The figure shows three views and two pictorial views of one solid part (mm, origin at its lowest corner). Answer the questions. A direction names the side the tool comes from. Coordinates: 2 decimals unless noted, no trailing zeros. Write each loop counter-clockwise with the first axis right and the second up, starting at its lowest first coordinate (ties: lowest second). Pieces come first, ordered by that corner, then holes.
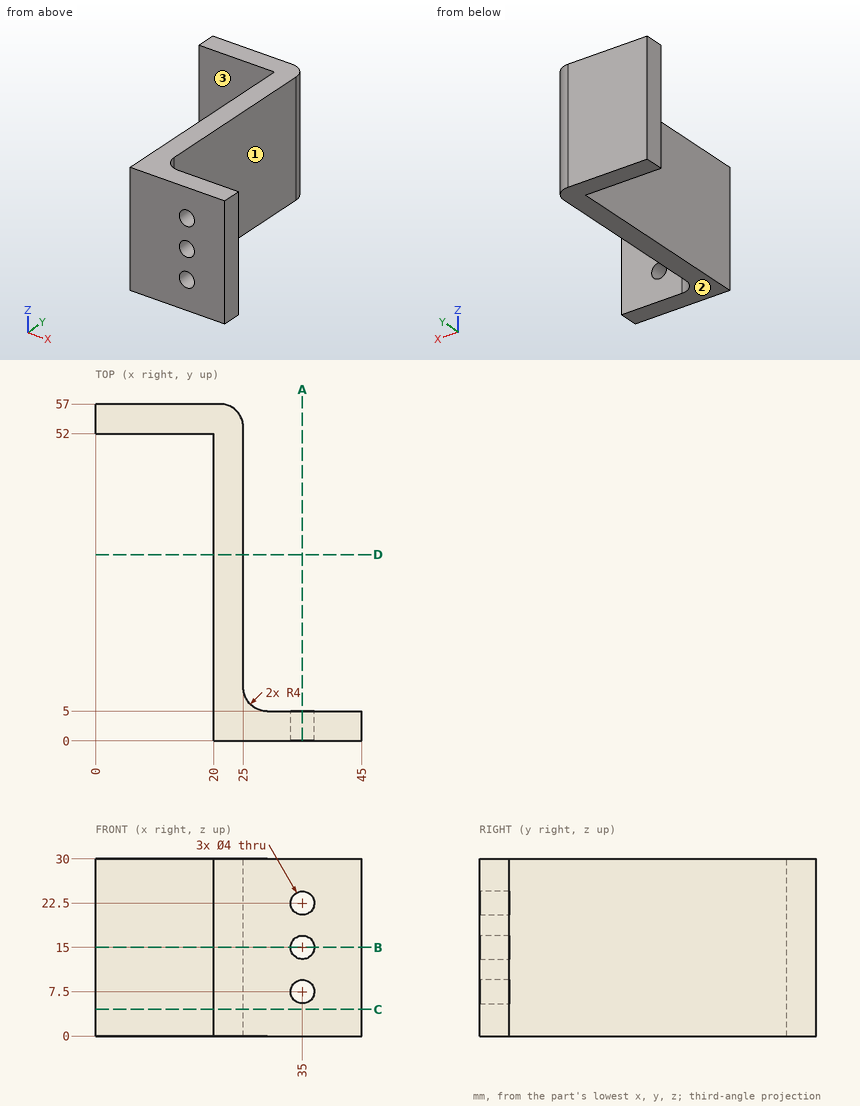
1. Section A-A on x = 35 is taken. Give the vertices of the cut face in (y, z).
Results found:
outline: (0, 0) - (5, 0) - (5, 5.5) - (0, 5.5) - close; (0, 9.5) - (5, 9.5) - (5, 13) - (0, 13) - close; (0, 17) - (5, 17) - (5, 20.5) - (0, 20.5) - close; (0, 24.5) - (5, 24.5) - (5, 30) - (0, 30) - close
2. Flat-ended cylindrical pins translate along their axes: P1, Ø5, axis at y = 48.5, z = 19.5, coming from the +X side; P2, Ø17.5, axis at x = 36, z = 20.5, coming from the +Y side; P3, Ø10, axis at x = 9, z = 17, coming from the -Y side. Find the tip coordinate at first contact, or state that the pin passes through.
Results found:
P1: stops at x = 25
P2: stops at y = 5.4
P3: stops at y = 52
3. Section D-D on y = 31.5 is taken. Give the vertices of the cut face in (x, z), then the cut area to 3 significant figures.
Results found:
outline: (20, 0) - (25, 0) - (25, 30) - (20, 30) - close
area: 150 mm2
4. Section B-B on z = 15 is taken. Give the vertices of the cut face in (x, y).
Results found:
outline: (0, 52) - (20, 52) - (20, 0) - (33, 0) - (33, 5) - (29, 5) arc R4 cw to (25, 9) - (25, 53) arc R4 ccw to (21, 57) - (0, 57) - close; (37, 0) - (45, 0) - (45, 5) - (37, 5) - close
5. Section C-C on z = 4.5 is taken. Give the vertices of the cut face in (x, y), then the cut area to 3 significant figures.
Results found:
outline: (0, 52) - (20, 52) - (20, 0) - (45, 0) - (45, 5) - (29, 5) arc R4 cw to (25, 9) - (25, 53) arc R4 ccw to (21, 57) - (0, 57) - close
area: 485 mm2
6. Find the intervals of material crossed by L1, parallel to X at y = 3.65, z = 15; L2, parallel to X at y = 24, z = 8.5; L3, parallel to Y at x = 14.5, z = 22, in increasing order.
Results found:
L1: x = 20 to 33, 37 to 45
L2: x = 20 to 25
L3: y = 52 to 57
7. A tool of negligible diameter and unlimited length cuts with its end or side. For the marked faces 1, 2 and 3, from which of +Z, -Z, +X, -X, +Y, -Y can it reach the whole face along a straight path? Write none if from no direction.
Results found:
face 1: +Z, -Z, +X, +Y
face 2: -Z, +X, -X, +Y, -Y
face 3: +Z, -Z, -X, -Y
